Check sheet for the drawn part. Datum: minimum x, y, z corner. Units: mm. Coordinates: 2 decimals unless noted, no trailing zeros. Loops run counter-clockwise (first coordinate to the right, second up) from the corner with the lowest first, then second, coordinate; pieces in that order, holes last.
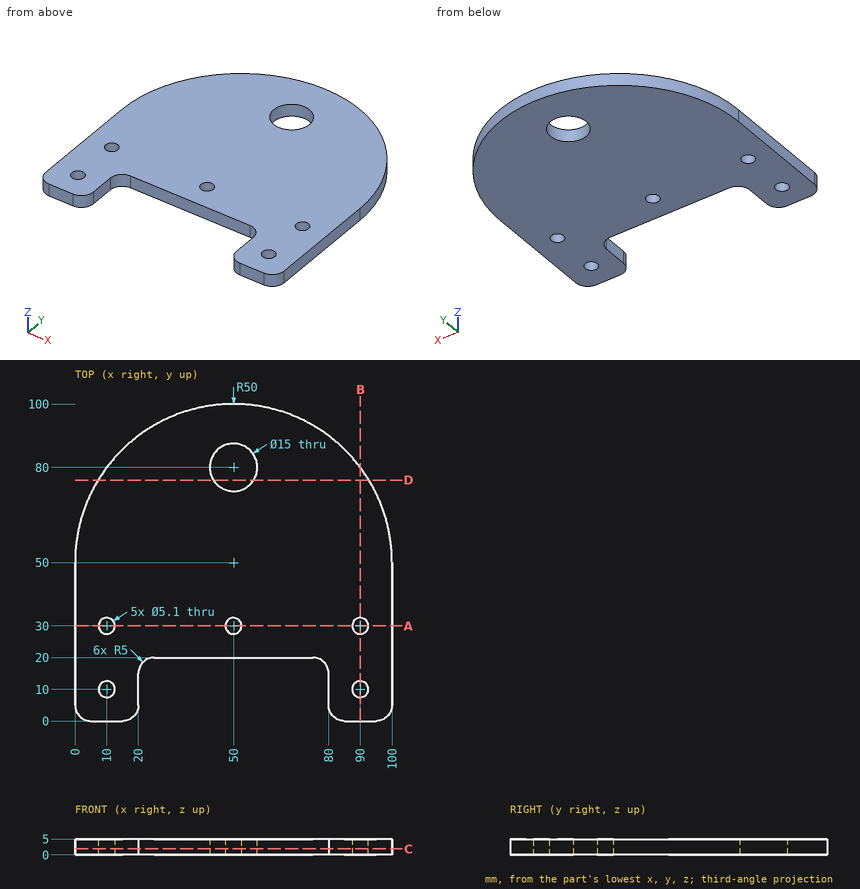
(1) Sectioned sample at A-A on y = 30. Record the cut outline in (x, z).
Findings:
outline: (0, 0) - (7.45, 0) - (7.45, 5) - (0, 5) - close; (12.55, 0) - (47.45, 0) - (47.45, 5) - (12.55, 5) - close; (52.55, 0) - (87.45, 0) - (87.45, 5) - (52.55, 5) - close; (92.55, 0) - (100, 0) - (100, 5) - (92.55, 5) - close
(2) Sectioned sample at C-C on z = 1.9. Record the cut outline in (x, y).
Findings:
outline: (0, 5) arc R5 ccw to (5, 0) - (15, 0) arc R5 ccw to (20, 5) - (20, 15) arc R5 cw to (25, 20) - (75, 20) arc R5 cw to (80, 15) - (80, 5) arc R5 ccw to (85, 0) - (95, 0) arc R5 ccw to (100, 5) - (100, 50) arc R50 ccw to (0, 50) - close; hole circle Ø5.1 at (10, 10); hole circle Ø5.1 at (10, 30); hole circle Ø15 at (50, 80); hole circle Ø5.1 at (50, 30); hole circle Ø5.1 at (90, 10); hole circle Ø5.1 at (90, 30)
(3) Gauge pin test, flat ends, axial feed: pin 1 Ø4.5 at (x, y) = (10, 30) entering from +Z; pin 2 Ø3 at (y, z) = (85, 4.5) entering from +X; pin 3 Ø2.5 at (x, z) = (62, 3.5) entering from -Y. Record the tip position at first contact, or that the pin passes through.
Findings:
pin 1: passes through
pin 2: stops at x = 87.12
pin 3: stops at y = 20
(4) Sectioned sample at D-D on y = 76. Record the cut outline in (x, z), and give its area (3 significant figures).
Findings:
outline: (7.29, 0) - (43.66, 0) - (43.66, 5) - (7.29, 5) - close; (56.34, 0) - (92.71, 0) - (92.71, 5) - (56.34, 5) - close
area: 364 mm2
(5) Scan lines: L1, parallel to Y at x = 90, z = 1.15; L2, parallel to Y at x = 50, z = 1.5; L3, parallel to X at y = 86.5, z = 3.9. Record each from-to range of solid material in increasing order.
Findings:
L1: y = 0 to 7.45, 12.55 to 27.45, 32.55 to 80
L2: y = 20 to 27.45, 32.55 to 72.5, 87.5 to 100
L3: x = 15.83 to 46.26, 53.74 to 84.17
(6) Sectioned sample at B-B on x = 90. Record the cut outline in (y, z), and give its area (3 significant figures).
Findings:
outline: (0, 0) - (7.45, 0) - (7.45, 5) - (0, 5) - close; (12.55, 0) - (27.45, 0) - (27.45, 5) - (12.55, 5) - close; (32.55, 0) - (80, 0) - (80, 5) - (32.55, 5) - close
area: 349 mm2
